from build123d import *

# Parameters (mm, degrees)
F1_DEPTH = 25
F2_R     = 4.473976
F3_DEPTH = 8


with BuildPart() as f1:
    # F0 (on Top) → F1 (new body)
    with BuildSketch(Plane.XY):
        with BuildLine():
            ThreePointArc((9.682585, -2.499508), (9.920329, -1.259791), (10, 0))
            ThreePointArc((10, 0), (9.920329, 1.259791), (9.682585, 2.499508))
            Line((9.682585, 2.499508), (-9.682585, 2.499508))
            ThreePointArc((-9.682585, 2.499508), (-10, 0), (-9.682585, -2.499508))
            Line((-9.682585, -2.499508), (9.682585, -2.499508))
        make_face()
    extrude(amount=F1_DEPTH)

    # F2 (on face) → F3 (join)
    with BuildSketch(Plane.XZ.offset(2.499508)):
        with Locations((0, 18.997351)):
            Circle(F2_R)
    extrude(amount=F3_DEPTH)


solid = f1.part
Part model, mm, in its own coordinate system. A direction names the side the tool comes from. Coordinates: 2 decimals unless noted, no trailing zeros. Loops run counter-clockwise (first coordinate to the right, second up) from the corner with the lowest first, then second, coordinate; pieces in that order, holes last. Notation, with made-up numbers: (-30.5, 4.25) - (24.5, 4.25) arc R26 ccw to (24.5, 37.25) - close; hole circle Ø10 at (49, 76.5). An arc over 180 degrees is marked (long way). Write each question's results on one line, items separated by ' | '. Start each with the question number.
Q1. Slice it at A-A on z = 9. Give the cut face in (x, y).
Q2. Which spindle directions (+Z, -Z, +X, -X, +Y, -Y) get a long thin tool onto all of the face, cutting with end or side? Do faces 1 (the cylindrical face through (-0.582, -6.444, 23.433)), 2 (the cylindrical face through (-10, 0, 12)). Say none if no direction does.
Q3. Probe line 1 along Y through (x, z) = (6.25, 18); line 2 along X through (y, z) = (-6, 18.75); line 3 along Z through (x, y) = (-0.25, -5.5). List the from-to ranges inside material, lowest first.
Q4. Slice it at B-B on x = 0. Give the cut face in (y, z), and give its area (3 significant figures).
Q5. Drop flat-ended pins along their axis: pin 1 Ø5 at (y, z) = (-4, 16) entering from -X; pin 2 Ø2 at (y, z) = (-4, 7.5) entering from +X; pin 3 Ø2 at (y, z) = (-5.5, 21.5) entering from +X; pin 4 Ø10 at (x, z) = (5, 4) entering from -Y. Give the stop position or say it passes through.
Q6. Slice it at D-D on y = -3.75. Give the cut face in (x, z).
Q7. Slice it at C-C on x = 3.25. Give the cut face in (y, z), and give its area (3 significant figures).
Answer:
1) outline: (-9.68, -2.5) - (9.68, -2.5) arc R10 ccw to (10, 0) arc R10 ccw to (9.68, 2.5) - (-9.68, 2.5) arc R10 ccw to start
2) face 1: -Y | face 2: +Z, -Z, -X
3) line 1: y = -2.5 to 2.5 | line 2: x = -4.47 to 4.47 | line 3: z = 14.53 to 23.46
4) outline: (-10.5, 14.52) - (-2.5, 14.52) - (-2.5, 0) - (2.5, 0) - (2.5, 25) - (-2.5, 25) - (-2.5, 23.47) - (-10.5, 23.47) - close | area: 197 mm2
5) pin 1: stops at x = -9.89 | pin 2: passes through | pin 3: stops at x = 4.21 | pin 4: stops at y = -2.5
6) outline: circle Ø8.95 at (0, 19)
7) outline: (-10.5, 15.92) - (-2.5, 15.92) - (-2.5, 0) - (2.5, 0) - (2.5, 25) - (-2.5, 25) - (-2.5, 22.07) - (-10.5, 22.07) - close | area: 174 mm2
